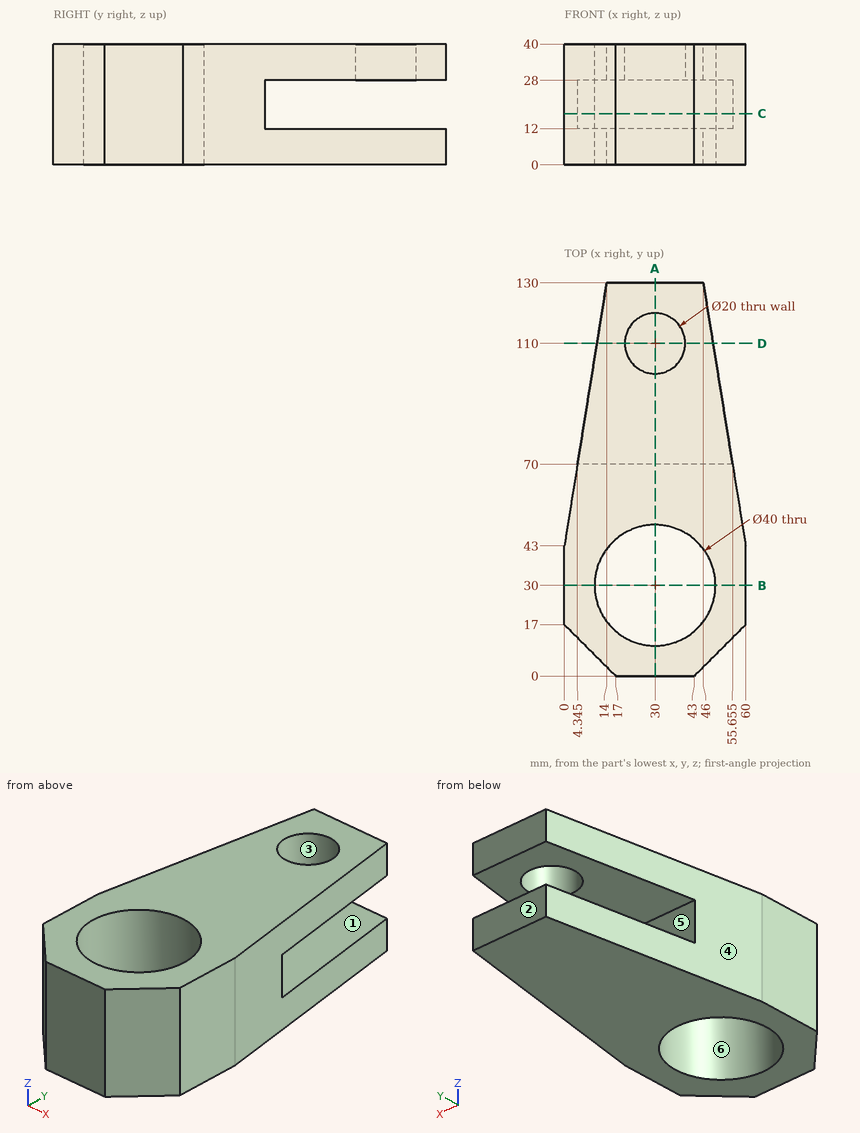
Design review of the part shown in the three views and the two pictorial views. Dimensions are in mm from the part's minimum x, y and z. A direction names the side the tool comes from. Round coordinates to 2 decimals unless told otherwise and drop trailing zeros. Order: outer loops, then holes, each group sorted by start corner. A loop starts at its lowest first (then second) coordinate and runs counter-clockwise, first axis right, second up. Notation, with made-up numbers: M 38,-38 L 46,-38 A18 ccw 46,-3 Z; hole C -29,0 d5. An arc over 180 degrees is marked long. Put each result on its own line as item: value.
Q1. Insertion check: pin 1 Ø8 at (x, z) = (17, 19.5) entering from +Y; pin 2 Ø3 at (y, z) = (88, 12) entering from +X; pin 3 Ø10 at (y, z) = (56.5, 19.5) entering from +X. Each pin has a flat end and moves straight along its axis. Give the tip position at first contact, or say it passes through.
Reported:
pin 1: y = 70
pin 2: x = 53
pin 3: x = 58.63
Q2. Consider section A-A (x = 30). State the section outline as (y, z) points.
Reported:
outline: M 0,0 L 10,0 L 10,40 L 0,40 Z; M 50,0 L 130,0 L 130,12 L 70,12 L 70,28 L 100,28 L 100,40 L 50,40 Z; M 120,28 L 130,28 L 130,40 L 120,40 Z
Q3. Consider section D-D (y = 110). State the section outline as (x, z) points.
Reported:
outline: M 10.78,0 L 49.22,0 L 49.22,12 L 10.78,12 Z; M 10.78,28 L 20,28 L 20,40 L 10.78,40 Z; M 40,28 L 49.22,28 L 49.22,40 L 40,40 Z
Q4. Draft analysis for pull direction X (two halves, no side actions). For the marked faces 4, 5 and 6, state which applies: released by +X, released by -X, zero draft, split by the parting line, or undercut.
Reported:
face 4: released by -X
face 5: zero draft
face 6: undercut
Q5. Consider section B-B (y = 30). State the section outline as (x, z) points, and give its area (3 significant figures).
Reported:
outline: M 0,0 L 10,0 L 10,40 L 0,40 Z; M 50,0 L 60,0 L 60,40 L 50,40 Z
area: 800 mm²
Q6. To check wall thickness, follow line 1 (Y direction, x = 30, z = 36); line 2 (Y direction, x = 30, z = 17); line 3 (Z direction, x = 23.5, y = 100.5). State the ranges of each line that lie inside material, in increasing order.
Reported:
line 1: 0 to 10, 50 to 100, 120 to 130
line 2: 0 to 10, 50 to 70
line 3: 0 to 12, 28 to 40
Q7. Machinability: for the marked faces 1, 2 and 3, which of the approach directions +Z, -Z, +X, -X, +Y, -Y give a long, thin tool a straight path to every point of the face, cutting with its end or side? Answer none if there is none.
Reported:
face 1: +X, -X, +Y
face 2: +Z, -Z, +X, -X, +Y
face 3: +Z
Q8. Consider section C-C (z = 17). State the section outline as (x, y) points (1 decimal), and give its area (3 significant figures).
Reported:
outline: M 0,17 L 17,0 L 43,0 L 60,17 L 60,43 L 55.7,70 L 4.3,70 L 0,43 Z; hole C 30,30 d40
area: 2,540 mm²
